```python
from build123d import *

# Parameters (mm, degrees)
F1_DEPTH  = 203.2
F2_T      = -6.35
F4_DEPTH  = 3.175
F5_W      = 292.1
F5_H      = 196.85
F6_DEPTH  = 640.08
F7_W      = 3.175
F7_H      = 254
F8_DEPTH  = 47.625
F10_W     = 3.175
F10_H     = 254
F11_DEPTH = 47.625
F12_DEPTH = 311.151


with BuildPart() as f1:
    # F0 (on Top) → F1 (new body)
    with BuildSketch(Plane.XY):
        Polygon((-168.573773, 0), (0, 0), (136.226227, 0), (136.226227, 355.6), (-168.573773, 355.6), align=None)
    extrude(amount=F1_DEPTH)

    # F2
    f2_openings = [f1.faces().sort_by_distance(p)[0] for p in [
        (-16.173773, 177.8, 0),
    ]]
    offset(amount=F2_T, openings=f2_openings)

    # F3 (on face) → F4 (join)
    with BuildSketch(Plane.XY.offset(203.2)):
        Polygon((-171.748773, 101.6), (-168.573773, 101.6), (-120.948773, 101.6), (-120.948773, 355.6), (-168.573773, 355.6), (-171.748773, 355.6), align=None)
        Polygon((139.401227, 355.6), (136.226227, 355.6), (88.601227, 355.6), (88.601227, 101.6), (136.226227, 101.6), (139.401227, 101.6), align=None)
    extrude(amount=F4_DEPTH)

    # F5 (on face) → F6 (cut)
    with BuildSketch(Plane.XZ):
        with Locations((-16.173773, 98.425)):
            Rectangle(F5_W, F5_H)
    extrude(amount=-F6_DEPTH, mode=Mode.SUBTRACT)

    # F7 (on face) → F8 (join)
    with BuildSketch(Plane(origin=(0, 0, 203.2), x_dir=(1, 0, 0), z_dir=(0, 0, -1))):
        with Locations((-170.161273, -228.6)):
            Rectangle(F7_W, F7_H)
    extrude(amount=F8_DEPTH)

    # F10 (on face) → F11 (join)
    with BuildSketch(Plane(origin=(0, 0, 203.2), x_dir=(1, 0, 0), z_dir=(0, 0, -1))):
        with Locations((137.813727, -228.6)):
            Rectangle(F10_W, F10_H)
    extrude(amount=F11_DEPTH)

    # F9 (on face) → F12 (cut, through all)
    with BuildSketch(Plane(origin=(-171.748773, 0, 0), x_dir=(0, -1, 0), z_dir=(-1, 0, 0))):
        with BuildLine():
            ThreePointArc((-287.3375, 180.975), (-292.1, 185.7375), (-296.8625, 180.975))
            Line((-296.8625, 180.975), (-287.3375, 180.975))
        make_face()
        with BuildLine():
            ThreePointArc((-160.3375, 180.975), (-165.1, 185.7375), (-169.8625, 180.975))
            Line((-169.8625, 180.975), (-160.3375, 180.975))
        make_face()
        with BuildLine():
            Line((-160.3375, 180.975), (-169.8625, 180.975))
            ThreePointArc((-169.8625, 180.975), (-165.1, 176.2125), (-160.3375, 180.975))
        make_face()
        with BuildLine():
            ThreePointArc((-223.8375, 180.975), (-228.6, 185.7375), (-233.3625, 180.975))
            Line((-233.3625, 180.975), (-223.8375, 180.975))
        make_face()
        with BuildLine():
            Line((-223.8375, 180.975), (-233.3625, 180.975))
            ThreePointArc((-233.3625, 180.975), (-228.6, 176.2125), (-223.8375, 180.975))
        make_face()
        with BuildLine():
            Line((-287.3375, 180.975), (-296.8625, 180.975))
            ThreePointArc((-296.8625, 180.975), (-292.1, 176.2125), (-287.3375, 180.975))
        make_face()
    extrude(amount=-F12_DEPTH, mode=Mode.SUBTRACT)


solid = f1.part
```
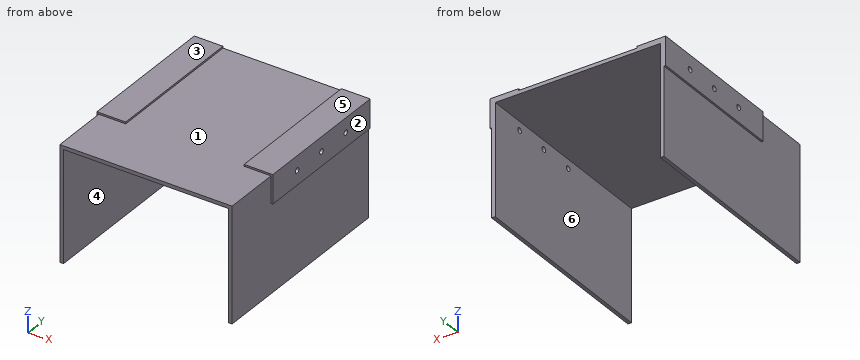
Part model, mm, in its own coordinate system. Face numbers are marked on the shaded views. A direction names the side the tool comes from. Coordinates: 2 decimals unless noted, no trailing zeros. Loops run counter-clockwise (first coordinate to the right, second up) from the corner with the lowest first, then second, coordinate; pieces in that order, holes last. Notation, with made-up numbers: (70, 38) - (99, 38) arc R18 cw to (99, 71) - close; hole circle Ø9 at (13, 29). An arc over 180 degrees is marked (long way). Write item = value, one per line. Start each with the question number.
Item 1: Mould opens along X. For the marked faces 1, 2, 3 and 4 say: released by +X, released by -X, zero draft, split by the parting line, or undercut.
Item 2: Cut at B-B, the plane z = 35. Give the cut face in (x, y), and give its area (3 significant figures).
Item 3: Cut at A-A, the plane y = 292.1. State how many separate pieces and enclosed holes the cut face has, and give its area (3 significant figures).
Item 4: Flat gauge pins, fed straight in: pin 1 Ø4 at (x, y) = (-105.5, 98) entering from +Z; pin 2 Ø8.5 at (y, z) = (165.1, 180.975) entering from -X; pin 3 Ø1.5 at (y, z) = (172, 38.5) entering from -X; pin 4 Ø1.5 at (y, z) = (313, 84.5) entering from +X. Where does each tip first touch, or does it go through?
Item 5: 3-axis set-ups, long thin cutter, end or side, ignore diameter. For the marked faces 5 and 6: which of +Z, -Z, +X, -X, +Y, -Y reach the whole face in a straight line?
Item 6: Cut at C-C, the plane x = 99. Give the cut face in (y, z) (3 decimals).
Item 7: Wall check: L1, parallel to X at y = 131.5, z = 182; L2, parallel to X at y = 252.5, z = 63; L3, parallel to Z at x = 136, y = 228 (3 decimals). Give the ranges that are in metal, low to high. Write a range as from..to.
Item 8: Cut at D-D, the plane y = 66. Give the cut face in (x, z).
The answers:
q1.face_1 = undercut
q1.face_2 = released by +X
q1.face_3 = zero draft
q1.face_4 = undercut
q2.outline = (-168.57, 0) - (-162.22, 0) - (-162.22, 355.6) - (-168.57, 355.6) - close; (129.88, 0) - (136.23, 0) - (136.23, 355.6) - (129.88, 355.6) - close
q2.area = 4,520 mm2
q3.separate_pieces = 3
q3.enclosed_holes = 0
q3.area = 4,880 mm2
q4.pin_1 = 203.2
q4.pin_2 = through
q4.pin_3 = -168.57
q4.pin_4 = 136.23
q5.face_5 = +Z, +X, -X, +Y, -Y
q5.face_6 = -Z, +Y, -Y
q6.outline = (0, 196.85) - (355.6, 196.85) - (355.6, 206.375) - (101.6, 206.375) - (101.6, 203.2) - (0, 203.2) - close
q7.L1 = -171.75..-162.22, 129.88..139.4
q7.L2 = -168.57..-162.22, 129.88..136.23
q7.L3 = 0..176.25, 185.7..206.375
q8.outline = (-168.57, 0) - (-162.22, 0) - (-162.22, 196.85) - (129.88, 196.85) - (129.88, 0) - (136.23, 0) - (136.23, 203.2) - (-168.57, 203.2) - close
